```python
from build123d import *


with BuildPart() as part:
    # Sketch1 → Revolve1 (revolve)
    with BuildSketch(Plane(origin=(0, 0, 0), x_dir=(1, 0, 0), z_dir=(0, 1, 0)), mode=Mode.PRIVATE) as revolve1_sk:
        Polygon((-28.5, 0), (28.5, 0), (28.5, 3.75), (28, 4.25), (26, 4.25), (25.5, 3.75), (25.5, 2.5), (-25.5, 2.5), (-25.5, 2.3), (-26.2, 2.3), (-26.2, 2.5), (-28, 2.5), (-28.5, 2), align=None)
    revolve(revolve1_sk.sketch.rotate(Axis((-28.5, 0, 0), (1, 0, 0)), 180), axis=Axis((-28.5, 0, 0), (1, 0, 0)))


solid = part.part
```
Model file for the job. Use its own axes, mm. A direction names the side the tool comes from. Coordinates: 2 decimals unless noted, no trailing zeros. Order: outer loops, then holes, each group sorted by start corner. A loop starts at its lowest first (then second) coordinate and runs counter-clockwise, first axis right, second up. Notation, with made-up numbers: M -35,60.5 L -3,60.5 A9 ccw -3,77.5 Z; hole C 18,18 d6. An arc over 180 degrees is marked long. Answer as CSV lines item,"result".
(1) 3-axis set-ups, long thin cutter, end or side, ignore diameter. For faces 1 (the cylindrical face through (-27.1, -0.1, -2.5)), 2 (the flat face through (-28.5, 0, 0)): which of +Z, -Z, +X, -X, +Y, -Y reach the whole face in a straight line?
Geometry says:
face 1,"-X"
face 2,"+Z, -Z, -X, +Y, -Y"
(2) Band-saw the part on C-C, the plane x = -24. List the corners of the cut face in (y, z).
Geometry says:
outline,"C 0,0 d5"
(3) Band-saw the part on A-A, the plane y = 0. List the corners of the cut face in (x, z).
Geometry says:
outline,"M -28.5,-2 L -28,-2.5 L -26.2,-2.5 L -26.2,-2.3 L -25.5,-2.3 L -25.5,-2.5 L 25.5,-2.5 L 25.5,-3.75 L 26,-4.25 L 28,-4.25 L 28.5,-3.75 L 28.5,3.75 L 28,4.25 L 26,4.25 L 25.5,3.75 L 25.5,2.5 L -25.5,2.5 L -25.5,2.3 L -26.2,2.3 L -26.2,2.5 L -28,2.5 L -28.5,2 Z"
(4) Flat gauge pins, fed straight in: pin 1 (1 mm diameter, centred on x = -1.5, y = 1.5, fed in from -Z); pin 2 (1.5 mm diameter, centred on y = -3, z = -2.5, fed in from -X); pin 3 (4 mm diameter, centred on x = 12, z = -1, fed in from +Y). Where does each tip first touch, or does it go through?
Geometry says:
pin 1,"stops at z = -2.29"
pin 2,"stops at x = 25.5"
pin 3,"stops at y = 2.5"
(5) Wall check: line 1 along X through (y, z) = (1, 3); line 2 along Z through (x, y) = (-1, 1); line 3 along Z through (x, y) = (-7, -1.5). Give the ranges that are in metal, low to high.
Geometry says:
line 1,"x = 25.5 to 28.5"
line 2,"z = -2.29 to 2.29"
line 3,"z = -2 to 2"
(6) Pull direction X, two halves, no side cores. Call faces 3 (the flat face through (25.5, -3, 0)), 4 (the cylindrical face through (26.986, -4.214, -0.553)), 5 (the cylindrical face through (-25.855, 1.4, -1.825)), 6 (the flat face through (28.5, 0, 0)): +X half, -X half, draft (parallel to the pull), parting line (faces both ways), or undercut.
Geometry says:
face 3,"-X half"
face 4,"draft"
face 5,"undercut"
face 6,"+X half"
